Autodesk Inventor part; units mm, degrees
ref_plane "YZ Plane" through (0, 0, 0) normal (1, 0, 0) x (0, 1, 0)
ref_plane "XZ Plane" through (0, 0, 0) normal (0, 1, 0) x (-1, 0, 0)
ref_plane "XY Plane" through (0, 0, 0) normal (0, 0, 1) x (1, 0, 0)
sketch "Sketch1" plane through (0, 0, 0) normal (0, 0, 1) x (1, 0, 0)
  line L0 (8.75, 10) -> (-8.75, 10)
  line L1 (-8.75, 10) -> (-8.75, -10)
  line L2 (-8.75, -10) -> (8.75, -10)
  line L3 (8.75, -10) -> (8.75, 10)
  line L4 (8.75, 10) -> (-8.75, -10) construction
  line L5 (-8.75, 10) -> (8.75, -10) construction
  line L6 (0, 10) -> (0, -10) construction
  line L7 (8.75, 0) -> (-8.75, 0) construction
  line L8 (0, -10) -> (0, 10) construction
  line L9 (0, -7.5) -> (0, 7.5) construction
  point P0 (0, 0)
  point P1 (0, 0)
  dimension "d0" = 17.5
  dimension "d1" = 20
  dimension "d19" = 15
extrude "Extrusion1" add sketch "Sketch1" along normal blind 1.6
hole "Phi2.5" at (0, -7.5, 0) at (0, 7.5, 0) direction (0, 0, 1) diameter 2.5 end through all
properties part number "SUSTAINA-SCI-EXTENSION-BORAD" material "CFRP"
Part model, mm, in its own coordinate system. Give positions to 0.01 mm unless a question says otherwise; leave off trailing zeros. Order: outer loops, then holes, each group sorted by start corner. A loop starts at its lowest first (then second) coordinate and runs counter-clockwise, first axis right, second up. Notation, with made-up numbers: M -19.75,12 L 5.25,12 A22 cw 5.25,20 Z; hole C 66.5,-2.5 d9. An arc over 180 degrees is marked long. Use a Markdown table: item, result. Add a question column.
(1) Saw through at B-B, the plane x = 0. Give the cut face in (y, z).
(2) Mould opens along X. For faces 1 (the face through (-0.05, 6.25, 0.81)), 2 (the face through (0, 0, 0)), 3 (the face through (8.75, 0, 1)) say: +X half, -X half, draft (parallel to the pull), parting line (faces both ways), or undercut.
(3) Saw through at A-A, the plane y = 6.75. Give the cut face in (x, z), and give its area (3 significant figures).
(4) Probe line 1 along Y through (x, z) = (0, 1.35); line 2 along X through (y, z) = (-7.5, 1.3); line 3 along Y through (x, z) = (-0.5, 0.55). List the from-to ranges inside material, lowest first. Write a range as [from, to].
(5) Saw through at C-C, the plane z = 1.1. Give the cut face in (x, y).
Answer key:
| question | item | result |
|---|---|---|
| 1 | outline | M -10,0 L -8.75,0 L -8.75,1.6 L -10,1.6 Z; M -6.25,0 L 6.25,0 L 6.25,1.6 L -6.25,1.6 Z; M 8.75,0 L 10,0 L 10,1.6 L 8.75,1.6 Z |
| 2 | face 1 | undercut |
| 2 | face 2 | draft |
| 2 | face 3 | +X half |
| 3 | outline | M -8.75,0 L -1,0 L -1,1.6 L -8.75,1.6 Z; M 1,0 L 8.75,0 L 8.75,1.6 L 1,1.6 Z |
| 3 | area | 24.8 mm^2 |
| 4 | line 1 | [-10, -8.75], [-6.25, 6.25], [8.75, 10] |
| 4 | line 2 | [-8.75, -1.25], [1.25, 8.75] |
| 4 | line 3 | [-10, -8.65], [-6.35, 6.35], [8.65, 10] |
| 5 | outline | M -8.75,-10 L 8.75,-10 L 8.75,10 L -8.75,10 Z; hole C 0,-7.5 d2.5; hole C 0,7.5 d2.5 |
